```python
from build123d import *

# Parameters (mm, degrees)
SKETCH_1_R           = 4.75
SKETCH_1_R_2         = 1.4
EXTRUDE_1_DEPTH      = 1.75
EXTRUDE_2_DEPTH      = 4.75
EXTRUDE_2_DEPTH_BACK = 4.75
SKETCH_3_R           = 1.4
CUT_EXTRUDE_1_DEPTH  = 71.22508455
FILLET_1_R           = 10
FILLET_2_R           = 10
SKETCH_5_W           = 18.718698013
SKETCH_5_H           = 4.522568897
CUT_EXTRUDE_3_DEPTH  = 71.796323339
CUT_EXTRUDE_4_DEPTH  = 53.363072215
CUT_EXTRUDE_5_DEPTH  = 53.363072215
SKETCH_10_W          = 0.8
SKETCH_10_H          = 4
EXTRUDE_3_DEPTH      = 3


with BuildPart() as part:
    # Sketch 1 → Extrude 1 (new body)
    with BuildSketch(Plane(origin=(0, 0, 0), x_dir=(1, 0, 0), z_dir=(0, 1, 0))):
        with Locations(Location((0, 0, 0), (0, 0, 270))):
            Circle(SKETCH_1_R)
        with Locations(Location((0, 0, 0), (0, 0, 270))):
            Circle(SKETCH_1_R_2, mode=Mode.SUBTRACT)
    extrude(amount=EXTRUDE_1_DEPTH)

    # Sketch 2 → Extrude 2 (add, two sides: drawn at the far end of the back side and taken through both)
    with BuildSketch(Plane.XY.offset(-EXTRUDE_2_DEPTH_BACK)):
        Polygon((14, 1.75), (50, 4.75), (70, 1.2), (70, 0), (65.316834236, 0), (48.921679528, 2.910139961), (14, 0), (0, 0), (0, 1.75), align=None)
    extrude(amount=EXTRUDE_2_DEPTH + EXTRUDE_2_DEPTH_BACK)

    # Sketch 3 → Cut-Extrude 1 (cut, through all)
    with BuildSketch(Plane(origin=(0, 1.75, 0), x_dir=(1, 0, 0), z_dir=(0, 1, 0))):
        with Locations(Location((0, 0, 0), (0, 0, 270))):
            Circle(SKETCH_3_R)
    extrude(amount=-CUT_EXTRUDE_1_DEPTH, mode=Mode.SUBTRACT)

    # Fillet 1
    fillet_1_edges = [part.edges().sort_by_distance(p)[0] for p in [
        (50, 4.75, 0),
        (48.921679528, 2.910139961, 0),
    ]]
    fillet(fillet_1_edges, radius=FILLET_1_R)

    # Fillet 2
    fillet_2_edges = [part.edges().sort_by_distance(p)[0] for p in [
        (65.316834236, 0, 0),
    ]]
    fillet(fillet_2_edges, radius=FILLET_2_R)

    # Sketch 5 → Cut-Extrude 3 (cut, through all)
    with BuildSketch(Plane.XY.offset(4.75)):
        with Locations((60.640650994, 2.261284449)):
            Rectangle(SKETCH_5_W, SKETCH_5_H)
    extrude(amount=-CUT_EXTRUDE_3_DEPTH, mode=Mode.SUBTRACT)

    # Sketch 6 → Cut-Extrude 4 (cut, through all)
    with BuildSketch(Plane.XY.offset(4.75)):
        with BuildLine():
            Line((51.281301987, 4.522568897), (51.281301987, 3.662250428))
            ThreePointArc((51.281301987, 3.662250428), (51.022669477, 4.326231546), (50.383057367, 4.640330335))
            ThreePointArc((50.383057367, 4.640330335), (50.833513908, 4.591626686), (51.281301987, 4.522568897))
        make_face()
    extrude(amount=-CUT_EXTRUDE_4_DEPTH, mode=Mode.SUBTRACT)

    # Sketch 7 → Cut-Extrude 5 (cut, through all)
    with BuildSketch(Plane.XY.offset(4.75)):
        with BuildLine():
            Line((51.281301987, 2.491306974), (51.281301987, 3.662250428))
            ThreePointArc((51.281301987, 3.662250428), (50.938888433, 2.917268377), (50.150530669, 2.692018883))
            Line((50.150530669, 2.692018883), (50.202981515, 2.682708858))
            Line((50.202981515, 2.682708858), (51.281301987, 2.491306974))
        make_face()
    extrude(amount=-CUT_EXTRUDE_5_DEPTH, mode=Mode.SUBTRACT)

    # Sketch 10 → Extrude 3 (add)
    with BuildSketch(Plane.XZ):
        with Locations((7.4, -2.75)):
            Rectangle(SKETCH_10_W, SKETCH_10_H)
    extrude(amount=EXTRUDE_3_DEPTH)

    # Mirror 1: part across plane


with BuildPart() as part_1:
    add(part.part)
    add(part.part.mirror(Plane.ZX.offset(-3)))


solid = part_1.part
```
Geometry check sheet. Reference: the model listing, model coordinates, mm. A direction names the side the tool comes from. Coordinates: 2 decimals unless noted, no trailing zeros. Order: outer loops, then holes, each group sorted by start corner. A loop starts at its lowest first (then second) coordinate and runs counter-clockwise, first axis right, second up. Notation, with made-up numbers: M -16,-15.5 L 19,-15.5 A14 ccw 19,-9.5 Z; hole C 19,45 d1. An arc over 180 degrees is marked long. One line per question, with ' | ' between items. Start each with the question number.
Item 1: Gauge pin test, flat ends, axial feed: pin 1 (5 mm diameter, centred on x = 7, z = 1.5, fed in from +Y); pin 2 (2 mm diameter, centred on y = 0.5, z = -3, fed in from -X); pin 3 (2 mm diameter, centred on x = 0, z = 0, fed in from -Y); pin 4 (5 mm diameter, centred on x = 0.5, z = 2, fed in from -Y). Record the tip position at first contact, or that the pin passes through.
Item 2: Set-up check for faces 4 (the flat face through (24, -7, -4.75)), 5 (the flat face through (7.8, -3, -3)), 6 (the flat face through (4, -7.75, 0)), 7 (the flat face through (26, 2, 4.75)), 8 (the cylindrical face through (48.9, 2.827, 0.067)): record each of +Z, -Z, +X, -X, +Y, -Y from which the full face is reachable in a straight line by a thin tool's end or side.
Item 3: Cross-section at B-B on y = 1. Enter the section's corners in (x, z).
Item 4: Draft check along Y on faces 1 (the flat face through (31.109, 3.176, -0.067)), 2 (the cylindrical face through (-4.75, -6.86, -0.1)), 3 (the flat face through (5, -6, 0)). Enter one of: pulls with the +Y half, pulls with the -Y half, needs draft (parallel to the pull), parting line crosses it, or undercut.
Item 5: Cross-section at A-A on z = 0. Enter the section's corners in (x, y), then the cut area to 3 significant figures.
Item 6: Material ranges on L1, parallel to Z at x = 0, y = 0.65; L2, parallel to Y at x = 13, z = 4; L3, parallel to Y at x = 27.5, z = 2.75 (3 decimals), recorded low to high. Write a range as [from, to].
Item 7: Cross-section at D-D on x = 40. Enter the section's corners in (y, z).
Item 8: Cross-section at C-C on z = 3.25. Enter the section's corners in (x, y), then the cut area to 3 significant figures.
Findings:
1) pin 1: stops at y = 1.75 | pin 2: stops at x = -4.31 | pin 3: passes through | pin 4: stops at y = -7.75
2) face 4: -Z, +X, -X, +Y, -Y | face 5: +Z, -Z, +X | face 6: +Z, -Z, -X, -Y | face 7: +Z, +X, -X, +Y, -Y | face 8: +Z, -Z
3) outline: M 0,-4.75 L 26,-4.75 L 26,4.75 L 0,4.75 A4.75 ccw Z; hole C 0,0 d2.8
4) face 1: pulls with the +Y half | face 2: needs draft | face 3: undercut
5) outline: M -4.75,-7.75 L -1.4,-7.75 L -1.4,-6 L -4.75,-6 Z; M -4.75,0 L -1.4,0 L -1.4,1.75 L -4.75,1.75 Z; M 1.4,-7.75 L 14,-7.75 L 48.7,-10.64 A10 ccw 50.38,-10.64 A0.98 ccw long 50.15,-8.69 L 50.2,-8.68 A10 cw 47.62,-8.8 L 14,-6 L 1.4,-6 Z; M 1.4,0 L 14,0 L 47.62,2.8 A10 cw 50.2,2.68 L 50.15,2.69 A0.98 ccw long 50.38,4.64 A10 ccw 48.7,4.64 L 14,1.75 L 1.4,1.75 Z | area: 186 mm²
6) L1: z = [-4.75, -1.4], [1.4, 4.75] | L2: y = [-7.75, -6], [0, 1.75] | L3: y = [-8.875, -7.125], [1.125, 2.875]
7) outline: M -9.92,-4.75 L -8.17,-4.75 L -8.17,4.75 L -9.92,4.75 Z; M 2.17,-4.75 L 3.92,-4.75 L 3.92,4.75 L 2.17,4.75 Z
8) outline: M -3.46,-7.75 L 14,-7.75 L 48.7,-10.64 A10 ccw 50.38,-10.64 A0.98 ccw long 50.15,-8.69 L 50.2,-8.68 A10 cw 47.62,-8.8 L 14,-6 L -3.46,-6 Z; M -3.46,0 L 14,0 L 47.62,2.8 A10 cw 50.2,2.68 L 50.15,2.69 A0.98 ccw long 50.38,4.64 A10 ccw 48.7,4.64 L 14,1.75 L -3.46,1.75 Z | area: 192 mm²
